The figure shows three views and two pictorial views of one solid part (mm, origin at its lowest corner). Answer the questions. A direction names the side the tool comes from. Coordinates: 2 decimals unless noted, no trailing zeros. Write each loop counter-clockwise with the first axis right and the second up, starting at its lowest first coordinate (ties: lowest second). Pieces come first, ordered by that corner, then holes. Notation, with made-up numbers: M 89,-4.5 L 116,-4.5 A33 cw 116,24.5 Z; hole C 52.5,83 d8. An arc over 180 degrees is marked long. Write item = value, one per line.
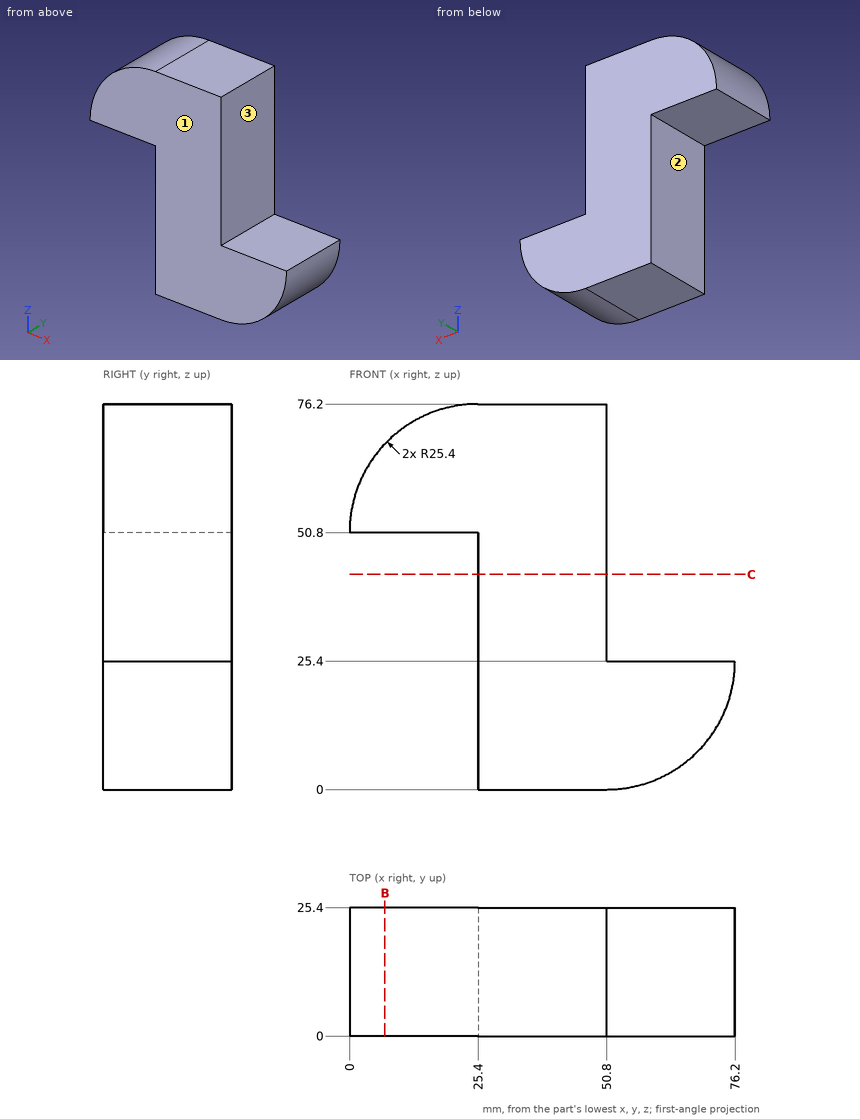
Item 1: Which of the six approach directions +Z, -Z, +X, -X, +Y, -Y give full straight-line access (tool end or side, diameter ignored) to the marked faces 1, 2 and 3?
Worked answers:
face_1 = +Z, -Z, +X, -X, -Y
face_2 = -Z, -X, +Y, -Y
face_3 = +Z, +X, +Y, -Y
Item 2: Consider line 1 along X through (y, z) = (2, 30); line 2 along X through (y, z) = (1, 58.5); line 3 along Z through (x, y) = (73, 13.75). Determine where each line is inside the solid, lowest interval first. Write a range as from..to.
Worked answers:
line_1 = 25.4..50.8
line_2 = 1.2..50.8
line_3 = 13.06..25.4
Item 3: Find section B-B (x = 7). Determine the outline of the cut face in (y, z).
Worked answers:
outline = M 0,50.8 L 25.4,50.8 L 25.4,68.31 L 0,68.31 Z
Item 4: Find section C-C (z = 42.5). Determine the outline of the cut face in (x, y).
Worked answers:
outline = M 25.4,0 L 50.8,0 L 50.8,25.4 L 25.4,25.4 Z
Item 5: Flat-ended cylindrical pins translate along their axes: pin 1 (1.5 mm diameter, centred on y = 12.5, z = 21.5, fed in from +X); pin 2 (4 mm diameter, centred on y = 3, z = 37, fed in from +X); pin 3 (5 mm diameter, centred on x = 12, y = 18.5, fed in from -Z). Find the tip coordinate at first contact, or state that the pin passes through.
Worked answers:
pin_1 = 76
pin_2 = 50.8
pin_3 = 50.8
